Input: part model. Units: mm. Frame: model coordinates. Give positions to 0.01 mm unless a question says otherwise; leave off trailing zeros. Loops run counter-clockwise (first coordinate to the right, second up) from the corner with the lowest first, then second, coordinate; pieces in that order, holes last. Notation, with made-up numbers: (24, 16.25) - (35, 16.25) arc R13 cw to (35, 40.25) - close; hole circle Ø5 at (19.5, -4.5). An arc over 180 degrees is marked (long way). One line per item, written item: value.
from build123d import *

# Parameters (mm, degrees)
SKETCH1_R           = 20.8
BOSS_EXTRUDE1_DEPTH = 5
SKETCH2_R           = 2.5
CUT_EXTRUDE1_DEPTH  = 381.250527306
SKETCH5_R           = 2.5
CUT_EXTRUDE5_DEPTH  = 209.206628137
FILLET1_R           = 0.4
FILLET2_R           = 3


with BuildPart() as part:
    # Sketch1 → Boss-Extrude1 (new body)
    with BuildSketch(Plane(origin=(0, 0, 0), x_dir=(1, 0, 0), z_dir=(0, 1, 0))):
        Polygon((0, -10), (190, -10), (190, 85), (0, 85), (-30, 85), (-30, -10), align=None)
        with Locations(Location((40, 37.5, 0), (0, 0, 270))):
            Circle(SKETCH1_R, mode=Mode.SUBTRACT)
    extrude(amount=BOSS_EXTRUDE1_DEPTH)

    # Sketch2 → Cut-Extrude1 (cut, through all)
    with BuildSketch(Plane(origin=(-147.27442804, 0, -165.531831037), x_dir=(1, 0, 0), z_dir=(0, -1, 0))):
        with Locations(Location((208.487631475, 149.245034473, 0), (0, 0, 270))):
            Circle(SKETCH2_R)
        with Locations(Location((208.487631475, 106.245034473, 0), (0, 0, 270))):
            Circle(SKETCH2_R)
        with Locations(Location((165.487631475, 149.245034473, 0), (0, 0, 270))):
            Circle(SKETCH2_R)
        with Locations(Location((165.487631475, 106.245034473, 0), (0, 0, 270))):
            Circle(SKETCH2_R)
    extrude(amount=-CUT_EXTRUDE1_DEPTH, mode=Mode.SUBTRACT)

    # Sketch5 → Cut-Extrude5 (cut, through all)
    with BuildSketch(Plane(origin=(0, 0, 0), x_dir=(-1, 0, 0), z_dir=(0, -1, 0))):
        with Locations(Location((21.499999973, 73, 0), (0, 0, 90))):
            Circle(SKETCH5_R)
        with Locations(Location((-46.160000027, 73, 0), (0, 0, 90))):
            Circle(SKETCH5_R)
        with Locations(Location((-113.820000027, 73, 0), (0, 0, 90))):
            Circle(SKETCH5_R)
        with Locations(Location((-181.480000027, 73, 0), (0, 0, 90))):
            Circle(SKETCH5_R)
        with Locations(Location((-181.480000027, 2, 0), (0, 0, 270))):
            Circle(SKETCH5_R)
        with Locations(Location((-113.820000027, 2, 0), (0, 0, 270))):
            Circle(SKETCH5_R)
        with Locations(Location((-46.160000027, 2, 0), (0, 0, 270))):
            Circle(SKETCH5_R)
        with Locations(Location((21.499999973, 2, 0), (0, 0, 270))):
            Circle(SKETCH5_R)
        with BuildLine():
            Line((20.499999973, 68.4), (22.499999973, 68.4))
            ThreePointArc((22.499999973, 68.4), (23.899999973, 67), (22.499999973, 65.6))
            Line((22.499999973, 65.6), (20.499999973, 65.6))
            ThreePointArc((20.499999973, 65.6), (19.099999973, 67), (20.499999973, 68.4))
        make_face()
        with BuildLine():
            Line((20.499999973, 81.7), (22.499999973, 81.7))
            ThreePointArc((22.499999973, 81.7), (23.799999973, 83), (22.499999973, 84.3))
            Line((22.499999973, 84.3), (22.499999973, 85))
            Line((22.499999973, 85), (20.499999973, 85))
            Line((20.499999973, 85), (20.499999973, 84.3))
            ThreePointArc((20.499999973, 84.3), (19.199999973, 83), (20.499999973, 81.7))
        make_face()
        with BuildLine():
            Line((-47.160000027, 68.4), (-45.160000027, 68.4))
            ThreePointArc((-45.160000027, 68.4), (-43.760000027, 67), (-45.160000027, 65.6))
            Line((-45.160000027, 65.6), (-47.160000027, 65.6))
            ThreePointArc((-47.160000027, 65.6), (-48.560000027, 67), (-47.160000027, 68.4))
        make_face()
        with BuildLine():
            Line((-47.160000027, 81.7), (-45.160000027, 81.7))
            ThreePointArc((-45.160000027, 81.7), (-43.860000027, 83), (-45.160000027, 84.3))
            Line((-45.160000027, 84.3), (-45.160000027, 85))
            Line((-45.160000027, 85), (-47.160000027, 85))
            Line((-47.160000027, 85), (-47.160000027, 84.3))
            ThreePointArc((-47.160000027, 84.3), (-48.460000027, 83), (-47.160000027, 81.7))
        make_face()
        with BuildLine():
            Line((-114.820000027, 68.4), (-112.820000027, 68.4))
            ThreePointArc((-112.820000027, 68.4), (-111.420000027, 67), (-112.820000027, 65.6))
            Line((-112.820000027, 65.6), (-114.820000027, 65.6))
            ThreePointArc((-114.820000027, 65.6), (-116.220000027, 67), (-114.820000027, 68.4))
        make_face()
        with BuildLine():
            Line((-114.820000027, 81.7), (-112.820000027, 81.7))
            ThreePointArc((-112.820000027, 81.7), (-111.520000027, 83), (-112.820000027, 84.3))
            Line((-112.820000027, 84.3), (-112.820000027, 85))
            Line((-112.820000027, 85), (-114.820000027, 85))
            Line((-114.820000027, 85), (-114.820000027, 84.3))
            ThreePointArc((-114.820000027, 84.3), (-116.120000027, 83), (-114.820000027, 81.7))
        make_face()
        with BuildLine():
            Line((-182.480000027, 68.4), (-180.480000027, 68.4))
            ThreePointArc((-180.480000027, 68.4), (-179.080000027, 67), (-180.480000027, 65.6))
            Line((-180.480000027, 65.6), (-182.480000027, 65.6))
            ThreePointArc((-182.480000027, 65.6), (-183.880000027, 67), (-182.480000027, 68.4))
        make_face()
        with BuildLine():
            Line((-182.480000027, 81.7), (-180.480000027, 81.7))
            ThreePointArc((-180.480000027, 81.7), (-179.180000027, 83), (-180.480000027, 84.3))
            Line((-180.480000027, 84.3), (-180.480000027, 85))
            Line((-180.480000027, 85), (-182.480000027, 85))
            Line((-182.480000027, 85), (-182.480000027, 84.3))
            ThreePointArc((-182.480000027, 84.3), (-183.780000027, 83), (-182.480000027, 81.7))
        make_face()
        with BuildLine():
            Line((-180.480000027, -10), (-182.480000027, -10))
            Line((-182.480000027, -10), (-182.480000027, -9.3))
            ThreePointArc((-182.480000027, -9.3), (-183.780000027, -8), (-182.480000027, -6.7))
            Line((-182.480000027, -6.7), (-180.480000027, -6.7))
            ThreePointArc((-180.480000027, -6.7), (-179.180000027, -8), (-180.480000027, -9.3))
            Line((-180.480000027, -9.3), (-180.480000027, -10))
        make_face()
        with BuildLine():
            Line((-112.820000027, -10), (-114.820000027, -10))
            Line((-114.820000027, -10), (-114.820000027, -9.3))
            ThreePointArc((-114.820000027, -9.3), (-116.120000027, -8), (-114.820000027, -6.7))
            Line((-114.820000027, -6.7), (-112.820000027, -6.7))
            ThreePointArc((-112.820000027, -6.7), (-111.520000027, -8), (-112.820000027, -9.3))
            Line((-112.820000027, -9.3), (-112.820000027, -10))
        make_face()
        with BuildLine():
            Line((-45.160000027, -10), (-47.160000027, -10))
            Line((-47.160000027, -10), (-47.160000027, -9.3))
            ThreePointArc((-47.160000027, -9.3), (-48.460000027, -8), (-47.160000027, -6.7))
            Line((-47.160000027, -6.7), (-45.160000027, -6.7))
            ThreePointArc((-45.160000027, -6.7), (-43.860000027, -8), (-45.160000027, -9.3))
            Line((-45.160000027, -9.3), (-45.160000027, -10))
        make_face()
        with BuildLine():
            Line((22.499999973, -10), (20.499999973, -10))
            Line((20.499999973, -10), (20.499999973, -9.3))
            ThreePointArc((20.499999973, -9.3), (19.199999973, -8), (20.499999973, -6.7))
            Line((20.499999973, -6.7), (22.499999973, -6.7))
            ThreePointArc((22.499999973, -6.7), (23.799999973, -8), (22.499999973, -9.3))
            Line((22.499999973, -9.3), (22.499999973, -10))
        make_face()
        with BuildLine():
            Line((-182.480000027, 6.6), (-180.480000027, 6.6))
            ThreePointArc((-180.480000027, 6.6), (-179.080000027, 8), (-180.480000027, 9.4))
            Line((-180.480000027, 9.4), (-182.480000027, 9.4))
            ThreePointArc((-182.480000027, 9.4), (-183.880000027, 8), (-182.480000027, 6.6))
        make_face()
        with BuildLine():
            Line((-114.820000027, 6.6), (-112.820000027, 6.6))
            ThreePointArc((-112.820000027, 6.6), (-111.420000027, 8), (-112.820000027, 9.4))
            Line((-112.820000027, 9.4), (-114.820000027, 9.4))
            ThreePointArc((-114.820000027, 9.4), (-116.220000027, 8), (-114.820000027, 6.6))
        make_face()
        with BuildLine():
            Line((-47.160000027, 6.6), (-45.160000027, 6.6))
            ThreePointArc((-45.160000027, 6.6), (-43.760000027, 8), (-45.160000027, 9.4))
            Line((-45.160000027, 9.4), (-47.160000027, 9.4))
            ThreePointArc((-47.160000027, 9.4), (-48.560000027, 8), (-47.160000027, 6.6))
        make_face()
        with BuildLine():
            Line((20.499999973, 6.6), (22.499999973, 6.6))
            ThreePointArc((22.499999973, 6.6), (23.899999973, 8), (22.499999973, 9.4))
            Line((22.499999973, 9.4), (20.499999973, 9.4))
            ThreePointArc((20.499999973, 9.4), (19.099999973, 8), (20.499999973, 6.6))
        make_face()
    extrude(amount=-CUT_EXTRUDE5_DEPTH, mode=Mode.SUBTRACT)

    # Fillet1
    # the kernel refuses this fillet: 0.4 mm, written as the material it takes off along each edge
    with BuildSketch(Plane(origin=(180.480000027, -0.88067791, 9.3), x_dir=(-0.9929562463235445, 0, -0.11848161413087033), z_dir=(0, 1, 0)), Plane(origin=(182.480000027, -0.88067791, -84.3), x_dir=(0.9929562463240562, 0, 0.11848161412658191), z_dir=(0, 1, 0)), Plane(origin=(45.160000027, -0.88067791, 9.3), x_dir=(-0.9929562463237254, 0, -0.11848161412935371), z_dir=(0, 1, 0)), Plane(origin=(112.820000027, -0.88067791, 9.3), x_dir=(-0.9929562463236348, 0, -0.11848161413011311), z_dir=(0, 1, 0)), Plane(origin=(-20.499999973, -0.88067791, -84.3), x_dir=(0.9929562463238144, 0, 0.11848161412860814), z_dir=(0, 1, 0)), Plane(origin=(47.160000027, -0.88067791, -84.3), x_dir=(0.9929562463238953, 0, 0.11848161412793001), z_dir=(0, 1, 0)), Plane(origin=(114.820000027, -0.88067791, -84.3), x_dir=(0.9929562463239765, 0, 0.11848161412724918), z_dir=(0, 1, 0)), Plane(origin=(-22.499999973, -0.88067791, 9.3), x_dir=(-0.9929562463238167, 0, -0.11848161412858836), z_dir=(0, 1, 0))) as fillet1_piece_1:
        with BuildLine():
            CenterArc((0.355444842, 0.397182499), FILLET1_R, 186.804480316, 76.391039369)
            Line((-0.041737656, 0.349789853), (0, 0))
            ThreePointArc((0, 0), (0.154026098, 0.00915688), (0.308052197, 0))
        make_face()
    extrude(amount=6.761355821, mode=Mode.SUBTRACT)
    with BuildSketch(Plane(origin=(180.480000027, -1, 10), x_dir=(0, 0, -1), z_dir=(0, 1, 0)), Plane(origin=(182.480000027, -1, 10), x_dir=(1, 0, 0), z_dir=(0, 1, 0)), Plane(origin=(180.480000027, -1, -85), x_dir=(-1, 0, 0), z_dir=(0, 1, 0)), Plane(origin=(45.160000027, -1, 10), x_dir=(0, 0, -1), z_dir=(0, 1, 0)), Plane(origin=(47.160000027, -1, 10), x_dir=(1, 0, 0), z_dir=(0, 1, 0)), Plane(origin=(112.820000027, -1, 10), x_dir=(0, 0, -1), z_dir=(0, 1, 0)), Plane(origin=(114.820000027, -1, 10), x_dir=(1, 0, 0), z_dir=(0, 1, 0)), Plane(origin=(-20.499999973, -1, -85), x_dir=(0, 0, 1), z_dir=(0, 1, 0)), Plane(origin=(-22.499999973, -1, -85), x_dir=(-1, 0, 0), z_dir=(0, 1, 0)), Plane(origin=(47.160000027, -1, -85), x_dir=(0, 0, 1), z_dir=(0, 1, 0)), Plane(origin=(45.160000027, -1, -85), x_dir=(-1, 0, 0), z_dir=(0, 1, 0)), Plane(origin=(114.820000027, -1, -85), x_dir=(0, 0, 1), z_dir=(0, 1, 0)), Plane(origin=(112.820000027, -1, -85), x_dir=(-1, 0, 0), z_dir=(0, 1, 0)), Plane(origin=(-22.499999973, -1, 10), x_dir=(0, 0, -1), z_dir=(0, 1, 0)), Plane(origin=(-20.499999973, -1, 10), x_dir=(1, 0, 0), z_dir=(0, 1, 0))) as fillet1_piece_2:
        with BuildLine():
            CenterArc((FILLET1_R, FILLET1_R), FILLET1_R, 180, 90)
            Line((0, FILLET1_R), (0, 0))
            Line((0, 0), (FILLET1_R, 0))
        make_face()
    extrude(amount=7, mode=Mode.SUBTRACT)
    with BuildSketch(Plane(origin=(182.480000027, -0.88067791, 9.3), x_dir=(0, 0, 1), z_dir=(0, 1, 0)), Plane(origin=(180.480000027, -0.88067791, -84.3), x_dir=(0, 0, -1), z_dir=(0, 1, 0)), Plane(origin=(47.160000027, -0.88067791, 9.3), x_dir=(0, 0, 1), z_dir=(0, 1, 0)), Plane(origin=(114.820000027, -0.88067791, 9.3), x_dir=(0, 0, 1), z_dir=(0, 1, 0)), Plane(origin=(-22.499999973, -0.88067791, -84.3), x_dir=(0, 0, -1), z_dir=(0, 1, 0)), Plane(origin=(45.160000027, -0.88067791, -84.3), x_dir=(0, 0, -1), z_dir=(0, 1, 0)), Plane(origin=(112.820000027, -0.88067791, -84.3), x_dir=(0, 0, -1), z_dir=(0, 1, 0)), Plane(origin=(-20.499999973, -0.88067791, 9.3), x_dir=(0, 0, 1), z_dir=(0, 1, 0))) as fillet1_piece_3:
        with BuildLine():
            CenterArc((0.352271164, 0.4), FILLET1_R, 193.608960631, 76.391039369)
            ThreePointArc((-0.036498522, 0.305882353), (-0.00915688, 0.154026098), (0, 0))
            Line((0, 0), (0.352271164, 0))
        make_face()
    extrude(amount=6.761355821, mode=Mode.SUBTRACT)
    with BuildSketch(Plane(origin=(182.480000027, -1, -85), x_dir=(1, 0, 0), z_dir=(0, 1, 0))) as fillet1_piece_4:
        with BuildLine():
            CenterArc((FILLET1_R, -FILLET1_R), FILLET1_R, 90, 90)
            Line((0, -FILLET1_R), (0, 0))
            Line((0, 0), (FILLET1_R, 0))
        make_face()
    extrude(amount=7, mode=Mode.SUBTRACT)

    # Fillet2
    fillet2_edges = [part.edges().sort_by_distance(p)[0] for p in [
        (-30, 2.5, -85),
        (190, 2.5, -85),
        (190, 2.5, 10),
        (-30, 2.5, 10),
    ]]
    fillet(fillet2_edges, radius=FILLET2_R)


solid = part.part
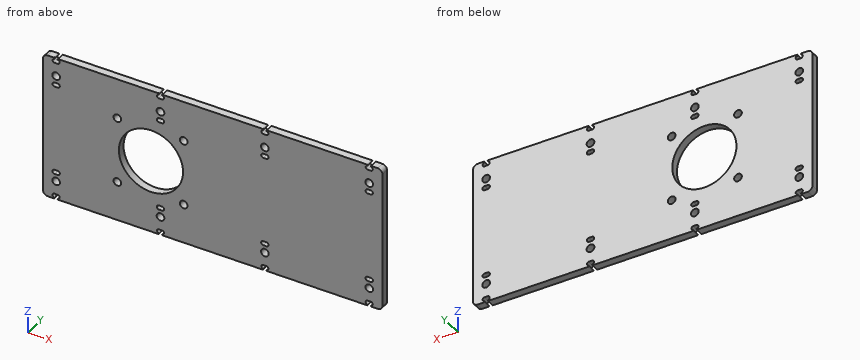
Item 1: Section A-A, the plane z = -37.5. Output: boundary loops of the cut face in (x, y), and give its area (3 significant figures).
Verdict:
outline: (-30, 0) - (19.2, 0) - (19.2, 5) - (-30, 5) - close; (60.8, 0) - (190, 0) - (190, 5) - (60.8, 5) - close
area: 892 mm^2
Item 2: Material intervals for L1, parallel to X at y = 2.15, z = -74; L2, parallel to Z at x = 19, y = 0.2; L3, parallel to X at y = 1.2, z = -66, sorted ascending.
Verdict:
L1: x = -30 to -23.79, -19.21 to 43.87, 48.45 to 111.53, 116.11 to 179.19, 183.77 to 190
L2: z = -85 to -61.66, -56.91 to -18.66, -13.91 to 10
L3: x = -30 to -23.48, -19.52 to 44.18, 48.14 to 111.84, 115.8 to 179.5, 183.46 to 190
Item 3: Pin query (flat end, axial travel): P1, Ø2, axis at x = 46.5, y = 2, coming from the +Z side; P2, Ø0.6, axis at x = 113.5, y = 3.5, coming from the +Z side; P3, Ø0.6, axis at x = 46, y = 1.5, coming from the -Z side. Return the tip coordinate at first contact, or that it passes through.
Verdict:
P1: stops at z = 10
P2: stops at z = 6.7
P3: stops at z = -81.7
Item 4: Section C-C, the plane x = 29. Output: boundary loops of the cut face in (y, z).
Verdict:
outline: (0, -85) - (5, -85) - (5, -55.15) - (0, -55.15) - close; (0, -19.85) - (5, -19.85) - (5, 10) - (0, 10) - close
Item 5: Section B-B, the plane z = -2. Output: boundary loops of the cut face in (x, y), and give its area (3 significant figures).
Verdict:
outline: (-30, 0) - (-24, 0) - (-24, 5) - (-30, 5) - close; (-19, 0) - (43.66, 0) - (43.66, 5) - (-19, 5) - close; (48.66, 0) - (111.32, 0) - (111.32, 5) - (48.66, 5) - close; (116.32, 0) - (178.98, 0) - (178.98, 5) - (116.32, 5) - close; (183.98, 0) - (190, 0) - (190, 5) - (183.98, 5) - close
area: 1,000 mm^2
Item 6: Section D-D, the plane z = -73.5. Output: boundary loops of the cut face in (x, y).
Verdict:
outline: (-30, 0) - (-23.95, 0) - (-23.95, 5) - (-30, 5) - close; (-19.05, 0) - (43.71, 0) - (43.71, 5) - (-19.05, 5) - close; (48.61, 0) - (111.37, 0) - (111.37, 5) - (48.61, 5) - close; (116.27, 0) - (179.03, 0) - (179.03, 5) - (116.27, 5) - close; (183.93, 0) - (190, 0) - (190, 5) - (183.93, 5) - close
